```python
from build123d import *

# Parameters (mm, degrees)
F1_DEPTH = 12.4968
F3_R     = 1.27
F4_DEPTH = 15.0114


with BuildPart() as f1:
    # F0 (on Top) → F1 (new body)
    with BuildSketch(Plane.XY):
        Polygon((25.8765831087, -15.494), (25.8765831087, 15.494), (-3.4604168913, 15.494), (-3.4604168913, 10.0838), (-18.4718168913, 10.0838), (-18.4718168913, -10.0838), (-3.4604168913, -10.0838), (-3.4604168913, -15.494), align=None)
        with BuildLine():
            ThreePointArc((4.3881831087, -13.6271), (2.7625831087, -12.0015), (4.3881831087, -10.3759))
            Line((4.3881831087, -10.3759), (8.8077831087, -10.3759))
            ThreePointArc((8.8077831087, -10.3759), (10.4333831087, -12.0015), (8.8077831087, -13.6271))
            Line((8.8077831087, -13.6271), (4.3881831087, -13.6271))
        make_face(mode=Mode.SUBTRACT)
        with BuildLine():
            ThreePointArc((4.4008831087, 10.3759), (2.7752831087, 12.0015), (4.4008831087, 13.6271))
            Line((4.4008831087, 13.6271), (8.8204831087, 13.6271))
            ThreePointArc((8.8204831087, 13.6271), (10.4460831087, 12.0015), (8.8204831087, 10.3759))
            Line((8.8204831087, 10.3759), (4.4008831087, 10.3759))
        make_face(mode=Mode.SUBTRACT)
    extrude(amount=F1_DEPTH)

    # F3
    f3_edges = [f1.edges().sort_by_distance(p)[0] for p in [
        (-3.460417, -15.494, 6.2484),
        (-3.460417, 15.494, 6.2484),
        (25.876583, -15.494, 6.2484),
        (25.876583, 15.494, 6.2484),
    ]]
    fillet(f3_edges, radius=F3_R)

    # F2 (on face) → F4 (cut)
    with BuildSketch(Plane(origin=(-18.4718168913, 0, 0), x_dir=(0, -1, 0), z_dir=(-1, 0, 0))):
        with BuildLine():
            Line((10.0838, 0), (10.0838, 6.2484))
            ThreePointArc((10.0838, 6.2484), (9.5260702319, 2.9412851884), (7.9145764182, 0))
            Line((7.9145764182, 0), (10.0838, 0))
        make_face()
        with BuildLine():
            ThreePointArc((7.9145764182, 12.4968), (9.5260702319, 9.5555148116), (10.0838, 6.2484))
            Line((10.0838, 6.2484), (10.0838, 12.4968))
            Line((10.0838, 12.4968), (7.9145764182, 12.4968))
        make_face()
        with BuildLine():
            ThreePointArc((-7.9145764182, 0), (0, -3.8354), (7.9145764182, 0))
            Line((7.9145764182, 0), (-7.9145764182, 0))
        make_face()
        with BuildLine():
            ThreePointArc((-10.0838, 6.2484), (-9.5260702319, 9.5555148116), (-7.9145764182, 12.4968))
            Line((-7.9145764182, 12.4968), (-10.0838, 12.4968))
            Line((-10.0838, 12.4968), (-10.0838, 6.2484))
        make_face()
        with BuildLine():
            Line((-10.0838, 0), (-7.9145764182, 0))
            ThreePointArc((-7.9145764182, 0), (-9.5260702319, 2.9412851884), (-10.0838, 6.2484))
            Line((-10.0838, 6.2484), (-10.0838, 0))
        make_face()
    extrude(amount=-F4_DEPTH, mode=Mode.SUBTRACT)


solid = f1.part
```
Input: part model. Units: mm. Frame: model coordinates. A direction names the side the tool comes from. Coordinates: 2 decimals unless noted, no trailing zeros. Loops run counter-clockwise (first coordinate to the right, second up) from the corner with the lowest first, then second, coordinate; pieces in that order, holes last. Notation, with made-up numbers: (19, -5.5) -> (38, -5.5) arc R17 ccw to (38, 12.5) -> close; hole circle Ø7 at (-16, -14.5). An arc over 180 degrees is marked (long way). Use a Markdown table: item, result.
1) Cut plane D-D (z = 1.5). Return the cut outline in (x, y), then the cut area to 3 significant figures.
Results found:
| item | result |
|---|---|
| outline | (-18.47, -8.9) -> (-3.46, -8.9) -> (-3.46, -14.22) arc R1.27 ccw to (-2.19, -15.49) -> (24.61, -15.49) arc R1.27 ccw to (25.88, -14.22) -> (25.88, 14.22) arc R1.27 ccw to (24.61, 15.49) -> (-2.19, 15.49) arc R1.27 ccw to (-3.46, 14.22) -> (-3.46, 8.9) -> (-18.47, 8.9) -> close; hole (4.39, -13.63) -> (8.81, -13.63) arc R1.63 ccw to (8.81, -10.38) -> (4.39, -10.38) arc R1.63 ccw to start; hole (4.4, 10.38) -> (8.82, 10.38) arc R1.63 ccw to (8.82, 13.63) -> (4.4, 13.63) arc R1.63 ccw to start |
| area | 1,130 mm2 |
2) Material intervals for line 1 along Y through (x, z) = (4.5, 2); line 2 along X through (y, z) = (-14, 6.75); line 3 along Y through (x, z) = (-6.5, 8.5), sorted ascending. Write a range as from..to.
Results found:
| item | result |
|---|---|
| line 1 | y = -15.49..-13.63, -10.38..10.38, 13.63..15.49 |
| line 2 | x = -3.46..25.88 |
| line 3 | y = -9.83..9.83 |
3) Access query for faces 1 (the flat face through (11, 15.494, 6)), 2 (the flat face through (7, -10.376, 6)). Directions: +Z, -Z, +X, -X, +Y, -Y. A direction counts if a zero-diameter tool reaches every point of the face in a straight line with its end or side. Return the directions, or none.
Results found:
| item | result |
|---|---|
| face 1 | +Z, -Z, +X, -X, +Y |
| face 2 | +Z, -Z |
4) Cut plane C-C (x = -12). Return the cut outline in (y, z), then the cut area to 3 significant figures.
Results found:
| item | result |
|---|---|
| outline | (-7.91, 0) -> (7.91, 0) arc R10.08 ccw to (7.91, 12.5) -> (-7.91, 12.5) arc R10.08 ccw to start |
| area | 235 mm2 |
5) Cut plane B-B (z = 10.25). Return the cut outline in (x, y).
Results found:
| item | result |
|---|---|
| outline | (-18.47, -9.26) -> (-3.46, -9.26) -> (-3.46, -14.22) arc R1.27 ccw to (-2.19, -15.49) -> (24.61, -15.49) arc R1.27 ccw to (25.88, -14.22) -> (25.88, 14.22) arc R1.27 ccw to (24.61, 15.49) -> (-2.19, 15.49) arc R1.27 ccw to (-3.46, 14.22) -> (-3.46, 9.26) -> (-18.47, 9.26) -> close; hole (4.39, -13.63) -> (8.81, -13.63) arc R1.63 ccw to (8.81, -10.38) -> (4.39, -10.38) arc R1.63 ccw to start; hole (4.4, 10.38) -> (8.82, 10.38) arc R1.63 ccw to (8.82, 13.63) -> (4.4, 13.63) arc R1.63 ccw to start |
6) Cut plane A-A (y = -12). Return the cut outline in (x, z).
Results found:
| item | result |
|---|---|
| outline | (-3.46, 0) -> (2.76, 0) -> (2.76, 12.5) -> (-3.46, 12.5) -> close; (10.43, 0) -> (25.88, 0) -> (25.88, 12.5) -> (10.43, 12.5) -> close |
7) Pull-direction query (Y, two-part tool) for faces 3 (the flat face through (11, -15.494, 6)), 4 (the flat face through (8, 0, 12.497)), 5 (the cylindrical face through (2.763, -12.037, 6.161)); classes: released by +Y, released by -Y, zero draft, split by the parting line, or undercut.
Results found:
| item | result |
|---|---|
| face 3 | released by -Y |
| face 4 | zero draft |
| face 5 | undercut |
